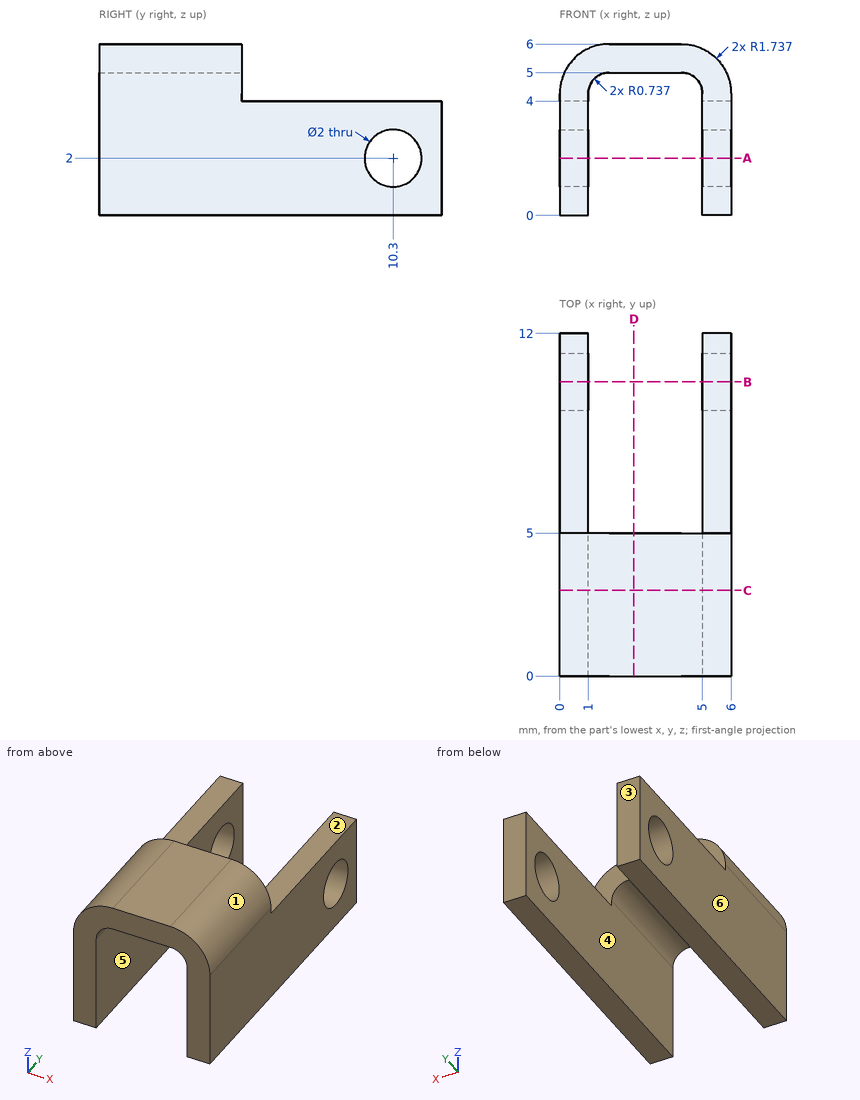
Study the drawing (mm; zero at the part's minimum x, y, z) and answer. A direction names the side the tool comes from. Coordinates: 2 decimals unless noted, no trailing zeros. Write each loop counter-clockwise with the first axis right and the second up, starting at its lowest first coordinate (ties: lowest second). Pieces come first, ordered by that corner, then holes. Notation, with made-up numbers: M 48,-23.5 L 84,-23.5 A20 cw 84,6.5 Z; hole C 19,36.25 d11. An arc over 180 degrees is marked long. Use one line per item in the form item = value.
Item 1: Find section A-A, the plane z = 2. Give the vertices of the cut face in (x, y).
Model answer:
outline = M 0,0 L 1,0 L 1,9.3 L 0,9.3 Z; M 0,11.3 L 1,11.3 L 1,12 L 0,12 Z; M 5,0 L 6,0 L 6,9.3 L 5,9.3 Z; M 5,11.3 L 6,11.3 L 6,12 L 5,12 Z
Item 2: Given P1, Ø1.6, axis at x = 2.5, z = 4.5, coming from the +Y side; P2, Ø0.5, axis at x = 5.5, y = 9.5, coming from the +Z side; P3, Ø1.5, axis at x = 5, y = 3, coming from the -Z side, each flat-ended and moving along its own axis, determine where each tip first touches the part or whether it passes through.
Model answer:
P1 = 5
P2 = 4
P3 = 0
Item 3: Find section D-D, the plane x = 2.6. Give the vertices of the cut face in (y, z).
Model answer:
outline = M 0,5 L 5,5 L 5,6 L 0,6 Z
Item 4: The mould has two halves that part along X. Classify the marked faces 3, 4, 5 and 6: released by +X, released by -X, zero draft, split by the parting line, or undercut.
Model answer:
face_3 = zero draft
face_4 = undercut
face_5 = undercut
face_6 = released by -X
Item 5: Find the intervals of material crossed by probe 1 along Y at (x, z) = (0.3, 2); probe 2 along X at (y, z) = (9.25, 1); probe 3 along Z at (x, y) = (3.95, 3), in increasing order.
Model answer:
probe_1 = 0 to 9.3, 11.3 to 12
probe_2 = 0 to 1, 5 to 6
probe_3 = 5 to 6
Item 6: Find section C-C, the plane y = 3. Give the vertices of the cut face in (x, z).
Model answer:
outline = M 0,0 L 1,0 L 1,4.26 A0.74 cw 1.74,5 L 4.26,5 A0.74 cw 5,4.26 L 5,0 L 6,0 L 6,4.26 A1.74 ccw 4.26,6 L 1.74,6 A1.74 ccw 0,4.26 Z
Item 7: For the marked faces 1 and 2, determine the directions among +Z, -Z, +X, -X, +Y, -Y from which every point of the face is accessible in a straight line to the end or side of a thin tool.
Model answer:
face_1 = +Z, +X, +Y, -Y
face_2 = +Z, +X, -X, +Y
Item 8: Find section B-B, the plane y = 10.3. Give the vertices of the cut face in (x, z).
Model answer:
outline = M 0,0 L 1,0 L 1,1 L 0,1 Z; M 0,3 L 1,3 L 1,4 L 0,4 Z; M 5,0 L 6,0 L 6,1 L 5,1 Z; M 5,3 L 6,3 L 6,4 L 5,4 Z
